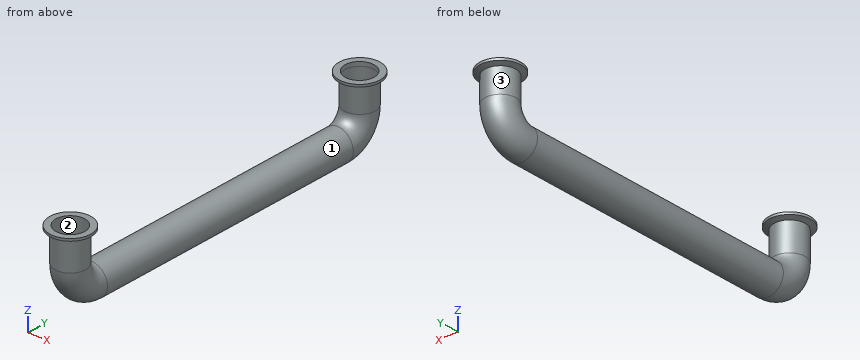
```python
from build123d import *

# Parameters (mm, degrees)
F2_R   = 19.05
F2_R_2 = 17.85


with BuildPart() as f1:
    # F0 (on Front) → F1 (revolve)
    with BuildSketch(Plane.XZ):
        Polygon((17.85, 5.1066154525), (17.85, 0), (19.05, 0), (25.25, 2.2566154525), (25.25, 5.1066154525), align=None)
    revolve(axis=Axis((0, 0, 5.6449943222), (0, 0, 1)))

    # F4: sweep along a path in F3
    with BuildLine(Plane.YZ) as f4_path:
        Line((0, 0), (0, -34.8933845475))
        ThreePointArc((0, -34.8933845475), (8.7867965644, -56.1065879831), (30, -64.8933845475))
        Line((30, -64.8933845475), (370, -64.8933845475))
        ThreePointArc((370, -64.8933845475), (391.2132034356, -56.1065879831), (400, -34.8933845475))
        Line((400, -34.8933845475), (400, -4.6830023639))
    # F2 (on Top) → F4 (sweep)
    with BuildSketch(Plane.XY):
        Circle(F2_R)
        Circle(F2_R_2, mode=Mode.SUBTRACT)
    sweep(path=f4_path.line)

    # F5 (on Right) → F6 (revolve)
    with BuildSketch(Plane.YZ):
        Polygon((417.85, 0.4236130886), (417.85, -4.6830023639), (419.05, -4.6830023639), (425.25, -2.4263869114), (425.25, 0.4236130886), align=None)
    revolve(axis=Axis((0, 400, -19.7881934557), (0, 0, 1)))


solid = f1.part
```
Work out the finished part from the listing and answer in its coordinate system (mm). Face numbers are marked on the shaded views. Give positions to 0.01 mm unless a question says otherwise; leave off trailing zeros. Loops run counter-clockwise (first coordinate to the right, second up) from the corner with the lowest first, then second, coordinate; pieces in that order, holes last. Notation, with made-up numbers: (56.5, 56.25) -> (90.5, 56.25) arc R8 ccw to (90.5, 64.25) -> close; hole circle Ø1 at (67, -37.75). An arc over 180 degrees is marked (long way). One line per question, with ' | ' between items. Start each with the question number.
1) Straight lines are drawn through the part: L1, parallel to Y at x = 0, z = -18; L2, parallel to Y at x = 0, z = -1.5; L3, parallel to X at y = 400, z = -13. For each, find the intervals that lie inside material, in ascending order.
2) Each of these flat-tipped pins is pushed along its axis until it touches: pin 1 (15 mm diameter, centred on x = -4.5, y = 410, fed in from +Z); pin 2 (6 mm diameter, centred on x = 11.5, z = -65.5, fed in from +Y); pin 3 (5 mm diameter, centred on x = -11.5, y = 357.5, fed in from +Z). Where does it stop, or does it pass through?
3) Determine the mould class of the marked faces 1, 2 and 3 for opening direction Z: +Z half, -Z half, draft (parallel to the pull), parting line (faces both ways), or undercut.
4) Section B-B, the plane z = -28 is taken. Determine the outline of the cut face in (x, y), then the cut area to 3 significant figures.
5) Section C-C, the plane y = 223.5 is taken. Determine the outline of the cut face in (x, z), then the cut area to 3 significant figures.
Resolved:
1) L1: -19.05 to -17.85, 17.85 to 19.05, 380.95 to 382.15, 417.85 to 419.05 | L2: -19.05 to -17.85, 17.85 to 19.05, 374.75 to 382.15, 417.85 to 425.25 | L3: -19.05 to -17.85, 17.85 to 19.05
2) pin 1: z = 0.42 | pin 2: y = 406.86 | pin 3: z = -48.1
3) face 1: parting line | face 2: draft | face 3: undercut
4) outline: circle Ø38.1 at (0, 0); circle Ø38.1 at (0, 400); hole circle Ø35.7 at (0, 0); hole circle Ø35.7 at (0, 400) | area: 278 mm2
5) outline: circle Ø38.1 at (0, -64.89); hole circle Ø35.7 at (0, -64.89) | area: 139 mm2
